Could you check a few things on this model? Use its own coordinates, in mm. Coordinates: 2 decimals unless noted, no trailing zeros. Loops run counter-clockwise (first coordinate to the right, second up) from the corner with the lowest first, then second, coordinate; pieces in that order, holes last. Notation, with made-up numbers: M -22,88 L 9,88 A28 cw 9,108 Z; hole C 6.25,61 d6. An arc over 180 degrees is marked long. Write each question's results on one line, items separated by ' | '.
Autodesk Inventor part; units mm, degrees
ref_plane "YZ Plane" through (0, 0, 0) normal (1, 0, 0) x (0, 1, 0)
ref_plane "XZ Plane" through (0, 0, 0) normal (0, 1, 0) x (-1, 0, 0)
ref_plane "XY Plane" through (0, 0, 0) normal (0, 0, 1) x (1, 0, 0)
sketch "Эскиз4" plane through (0, 0, 0) normal (1, 0, 0) x (0, 1, 0)
  line L0 (13.1772, 0) -> (-2.347, 0)
  line L1 (-2.347, 0) -> (-2.347, -10.7877)
  line L2 (-2.347, -10.7877) -> (13.1772, 0)
  point P0 (0, 0)
revolve "Вращение2" add sketch "Эскиз4" angle 360 about axis through (0, 13.1772, 0) along (0, -1, 0)
sketch "Эскиз5" plane through (0, 0, 0) normal (1, 0, 0) x (0, 1, 0)
  line L0 (13.1772, 0) -> (-2.347, -10.7877)
  line L1 (9.586, 3.1529) -> (6.8145, 3.1529)
  line L2 (6.8145, 3.1529) -> (6.8145, -4.4214)
  line L3 (6.8145, -4.4214) -> (9.586, -4.4214)
  line L4 (9.586, -4.4214) -> (9.586, 3.1529)
  point P0 (0, 0)
extrude "Выдавливание1" cut sketch "Эскиз5" against normal blind 4
properties part number "вырез"
(1) Will these pins go through, and if not, where does the flat tip stop? P1, Ø6, axis at x = -3.5, z = 2.5, coming from the +Y side; P2, Ø3, axis at x = 2, y = 3, coming from the +Z side; P3, Ø8, axis at y = 5, z = -7.5, coming from the +X side.
Reported:
P1: stops at y = 11.3 | P2: stops at z = 7.92 | P3: stops at x = 6.06
(2) Please list where these lines run through material, in increasing order: probe 1 along X at (y, z) = (6.25, -4.25); probe 2 along X at (y, z) = (5, -1.25); probe 3 along Y at (x, z) = (7.25, -5.25). Write a range as from..to.
Reported:
probe 1: x = -2.26..2.26 | probe 2: x = -5.54..5.54 | probe 3: y = -2.35..0.3
(3) If we mould it in two halves opening along Y, with no side actions, what happens to faces 1 (the conical face through (4.234, 7.031, 0.556)), 2 (the flat face through (-1, 8, 3.153)), 3 (the flat face through (0, -2.347, 0)), 4 (the flat face through (-1, 9.586, 0))? For each: released by +Y, released by -Y, zero draft, split by the parting line, or undercut.
Reported:
face 1: released by +Y | face 2: zero draft | face 3: released by -Y | face 4: undercut
(4) Imagine slicing it at B-B, the plane y = 1.25. List the corners of the cut face in (x, z) for me.
Reported:
outline: C 0,0 d16.58
(5) Imagine slicing it at A-A, the plane y = -1. List the corners of the cut face in (x, z) for me.
Reported:
outline: C 0,0 d19.7
